Job drawing, mm, ordinate dimensions from the low corner. One solid piece. A direction names the side the tool comes from. Round coordinates to 2 decimals unless told otherwise and drop trailing zeros. Loops run counter-clockwise (first coordinate to the right, second up) from the corner with the lowest first, then second, coordinate; pieces in that order, holes last.
1) Probe line 1 (X direction, y = 241.3, z = 6.5); line 2 (Y direction, x = 50.8, z = 3); line 3 (Z direction, x = 67.5, y = 27.5) (3 decimals). List the from-to ranges inside material, lowest first.
2) Band-saw the part on D-D, the plane y = 36. Write the cut outline in (x, z) (3 decimals), then the cut area to 3 significant figures.
3) Band-saw the part on C-C, the plane z = 4. Write the cut outline in (x, y), then the cut area to 3 significant figures.
4) Drop flat-ended pins along their axis: P1, Ø17.5, axis at y = 116.5, z = 29, coming from the +X side (3 decimals); P2, Ø7.5, axis at x = 12, z = 28, coming from the +Y side; P3, Ø12, axis at x = 51, y = 194.5, coming from the -Z side; P4, Ø10.5, axis at y = 253.5, z = 7, coming from the -X side. Give the stop position or say it passes through.
5) 3-axis set-ups, long thin cutter, end or side, ignore diameter. For the marked faces 1, 2 and 3: which of +Z, -Z, +X, -X, +Y, -Y reach the whole face in a straight line?
6) Band-saw the part on A-A, the plane y = 241.3. Write the cut outline in (x, z) (3 decimals), then the cut area to 3 significant figures.
7) Band-saw the part on B-B, the plane x = 50.8. Write the cut outline in (y, z) (3 decimals).
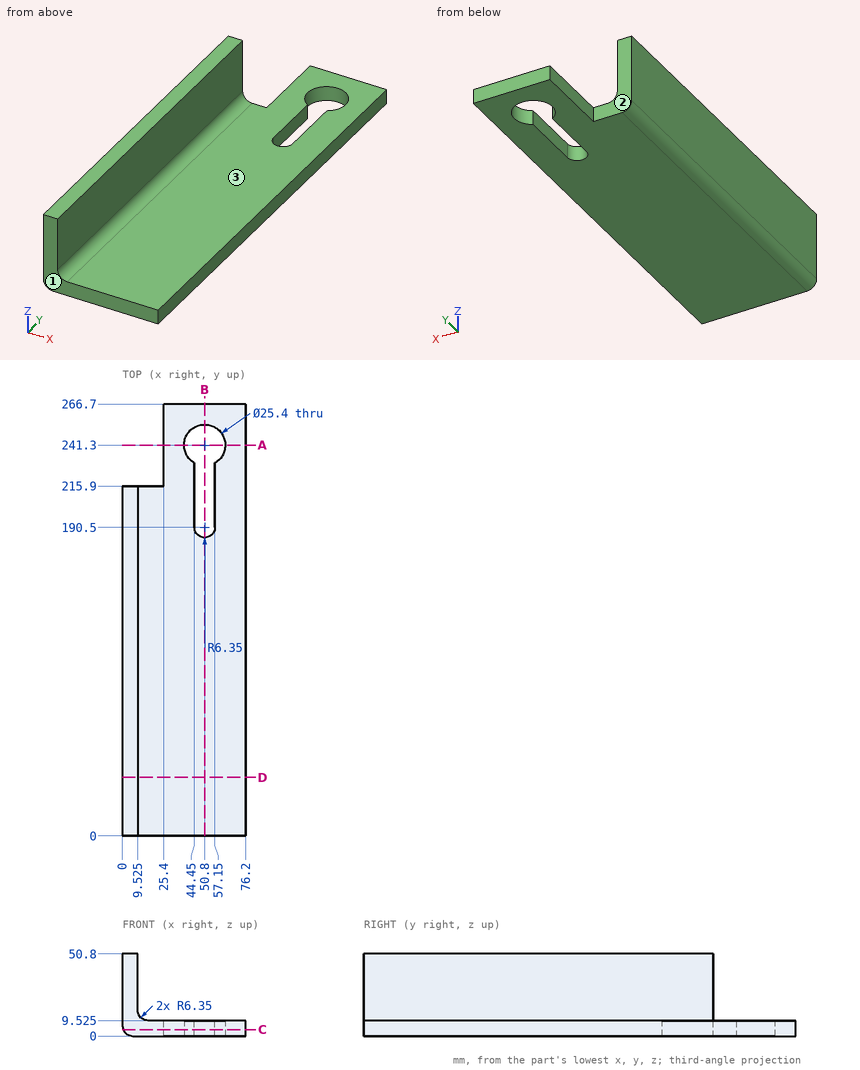
Reported:
1. line 1: x = 25.4 to 38.1, 63.5 to 76.2
1. line 2: y = 0 to 184.15, 254 to 266.7
1. line 3: z = 0 to 9.525
2. outline: (0, 6.35) arc R6.35 ccw to (6.35, 0) - (76.2, 0) - (76.2, 9.525) - (15.875, 9.525) arc R6.35 cw to (9.525, 15.875) - (9.525, 50.8) - (0, 50.8) - close
2. area: 1,120 mm2
3. outline: (0.45, 0) - (76.2, 0) - (76.2, 266.7) - (25.4, 266.7) - (25.4, 215.9) - (0.45, 215.9) - close; hole (44.45, 190.5) arc R6.35 ccw to (57.15, 190.5) - (57.15, 230.3) arc R12.7 ccw (long way) to (44.45, 230.3) - close
3. area: 17,900 mm2
4. P1: stops at x = 9.525
4. P2: stops at y = 215.9
4. P3: passes through
4. P4: stops at x = 25.4
5. face 1: +Z, -Z, +X, -X, -Y
5. face 2: +Z, -Z, -X, +Y
5. face 3: +Z, +X, +Y, -Y
6. outline: (25.4, 0) - (38.1, 0) - (38.1, 9.525) - (25.4, 9.525) - close; (63.5, 0) - (76.2, 0) - (76.2, 9.525) - (63.5, 9.525) - close
6. area: 242 mm2
7. outline: (0, 0) - (184.15, 0) - (184.15, 9.525) - (0, 9.525) - close; (254, 0) - (266.7, 0) - (266.7, 9.525) - (254, 9.525) - close
